Part model, mm, in its own coordinate system. A direction names the side the tool comes from. Give positions to 0.01 mm unless a question says otherwise; leave off trailing zeros. Write each loop counter-clockwise with the first axis right and the second up, starting at its lowest first coordinate (ties: lowest second). Pieces come first, ordered by that corner, then holes.
```python
from build123d import *

# Parameters (mm, degrees)
F0_W     = 850.9
F0_H     = 889
F0_W_2   = 774.7
F0_H_2   = 812.8
F1_DEPTH = 31.75
F2_W     = 19.05
F2_H     = 812.8
F3_DEPTH = 12.7
F5_DEPTH = 19.05


with BuildPart() as f1:
    # F0 (on Front) → F1 (new body)
    with BuildSketch(Plane.XZ):
        Rectangle(F0_W, F0_H)
        Rectangle(F0_W_2, F0_H_2, mode=Mode.SUBTRACT)
    extrude(amount=F1_DEPTH)

    # F2 (on face) → F3 (join)
    with BuildSketch(Plane(origin=(0, 0, 0), x_dir=(-1, 0, 0), z_dir=(0, 1, 0))):
        with Locations((-286.258, 0)):
            Rectangle(F2_W, F2_H)
        with Locations((-172.466, 0)):
            Rectangle(F2_W, F2_H)
        with Locations((-58.674, 0)):
            Rectangle(F2_W, F2_H)
        with Locations((55.118, 0)):
            Rectangle(F2_W, F2_H)
        with Locations((168.91, 0)):
            Rectangle(F2_W, F2_H)
        with Locations((282.702, 0)):
            Rectangle(F2_W, F2_H)
    extrude(amount=-F3_DEPTH)

    # F4 (on face) → F5 (join)
    with BuildSketch(Plane.XZ.offset(31.75)):
        Polygon((387.35, -373.689115), (-365.973302, 406.4), (-387.35, 406.4), (-387.35, 373.689115), (365.973302, -406.4), (387.35, -406.4), align=None)
    extrude(amount=-F5_DEPTH)


solid = f1.part
```
1) Saw through at B-B, the plane x = -233. Write the cut outline in (y, z), then the cut area to 3 significant figures.
Answers follow:
outline: (-31.75, -444.5) - (0, -444.5) - (0, -406.4) - (-31.75, -406.4) - close; (-31.75, 213.86) - (-12.7, 213.86) - (-12.7, 268.7) - (-31.75, 268.7) - close; (-31.75, 406.4) - (0, 406.4) - (0, 444.5) - (-31.75, 444.5) - close
area: 3,460 mm2
2) Pin check, flat tip, straight feed: pin 1 Ø21 at (x, z) = (-165.5, -180) entering from -Y. Stop position of the tip, or through.
Answers follow:
pin 1: stops at y = -12.7
3) Two-plate mould, pull along X, no slides. Class faces 1 (the face through (-6, -16, -444.5)), 2 (the face through (387.35, -16, -6)), 3 (the face through (-425.45, -16, -6)): +X half, -X half, draft (parallel to the pull), parting line (faces both ways), or undercut.
Answers follow:
face 1: draft
face 2: undercut
face 3: -X half
4) Wall check: L1, parallel to Z at x = -10, y = -10; L2, parallel to Z at x = 327, y = -14; L3, parallel to Z at x = 232.5, y = -15.5. Give the ranges that are in metal, low to high.
Answers follow:
L1: z = -444.5 to -406.4, 406.4 to 444.5
L2: z = -444.5 to -406.4, -366.04 to -311.19, 406.4 to 444.5
L3: z = -444.5 to -406.4, -268.18 to -213.34, 406.4 to 444.5
5) Saw through at A-A, the plane y = -6.5. Count the separate pieces of the cut face and the enclosed holes in it, then the cut area to 3 significant figures.
Answers follow:
separate pieces: 1
enclosed holes: 7
area: 220,000 mm2
6) 3-axis set-ups, long thin cutter, end or side, ignore diameter. For faces 4 (the face through (-55, -12.7, -180)), 5 (the face through (-112, -12.7, 116)), 6 (the face through (425.45, -16, -6)): which of +Z, -Z, +X, -X, +Y, -Y reach the whole face in a straight line?
Answers follow:
face 4: -Y
face 5: +Y
face 6: +Z, -Z, +X, +Y, -Y
